from build123d import *

# Parameters (mm, degrees)
REDONDEO1_R = 1


with BuildPart() as part:
    # Croquis1 → Revolución1 (revolve)
    with BuildSketch(Plane.XY, mode=Mode.PRIVATE) as revoluci_n1_sk:
        Polygon((0, 2.465), (9.82, 2.465), (9.82, 6.5), (3, 6.5), (3, 8), (0, 8), align=None)
    revolve(revoluci_n1_sk.sketch.rotate(Axis((0, 0, 0), (1, 0, 0)), 90), axis=Axis((0, 0, 0), (1, 0, 0)))

    # Redondeo1
    redondeo1_edges = [part.edges().sort_by_distance(p)[0] for p in [
        (0, 0, -8),
        (9.82, 0, -6.5),
    ]]
    fillet(redondeo1_edges, radius=REDONDEO1_R)


solid = part.part
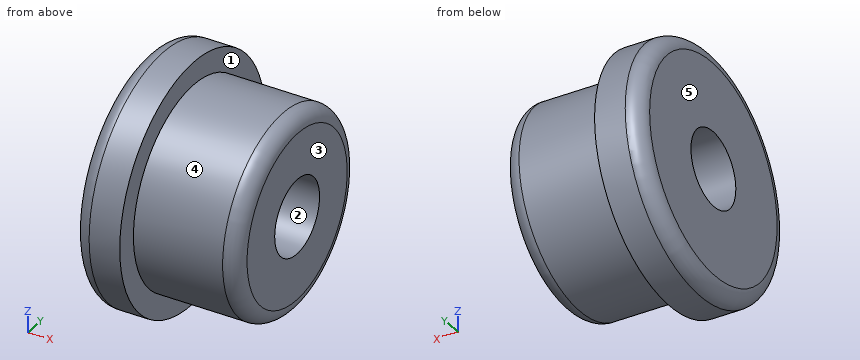
Geometry: final body of the model. Coordinates: model frame, mm. Face numbers are marked on the shaded views. A direction names the side the tool comes from. Coordinates: 2 decimals unless noted, no trailing zeros. Loops run counter-clockwise (first coordinate to the right, second up) from the corner with the lowest first, then second, coordinate; pieces in that order, holes last. Notation, with made-up numbers: M 61,-34 L 86,-34 A30 cw 86,-7 Z; hole C 21.25,80.25 d7. An arc over 180 degrees is marked long. One line per item, written item: value. Start each with the question number.
1) Cut plane A-A (z = 0). Return loops of the section in (x, y) (3 decimals).
2) Reachability of the marked faces 1 and 2 from +Z, -Z, +X, -X, +Y, -Y: full face, straight path, thin tool, end or side. Return the list, or none.
3) Pin query (flat end, axial travel): P1, Ø3, axis at y = 5, z = 1, coming from the -X side; P2, Ø4, axis at x = 6.5, z = -3, coming from the +Y side; P3, Ø1.5, axis at x = 8.5, y = -2.5, coming from the +Z side; P4, Ø4, axis at x = 3, y = -3.5, coming from the +Z side. Return the tip coordinate at first contact, or that it passes through.
4) Draft query along X for the marked faces 3, 4 and 5. Return one class per face: released by +X, released by -X, zero draft, split by the parting line, or undercut.
5) Cut plane C-C (x = 2.5). Return loops of the section in (y, z) (3 decimals), then the cut area to 3 significant figures.
6) Cut plane D-D (x = 0.5). Return loops of the section in (y, z) (3 decimals), then the cut area to 3 significant figures.
7) Material intervals for L1, parallel to Y at x = 7.25, z = 0 (3 decimals); L2, parallel to Y at x = 1.75, z = 0 (3 decimals); L3, parallel to X at y = 2.5, z = -5, sorted ascending. Write a range as from..to.
Evaluation:
1. outline: M 0,-7 A1 ccw 1,-8 L 3,-8 L 3,-6.5 L 8.82,-6.5 A1 ccw 9.82,-5.5 L 9.82,-2.465 L 0,-2.465 Z; M 0,2.465 L 9.82,2.465 L 9.82,5.5 A1 ccw 8.82,6.5 L 3,6.5 L 3,8 L 1,8 A1 ccw 0,7 Z
2. face 1: +X
2. face 2: +X, -X
3. P1: x = 0
3. P2: y = 6.42
3. P3: z = 6.26
3. P4: z = 7.86
4. face 3: released by +X
4. face 4: zero draft
4. face 5: released by -X
5. outline: C 0,0 d16; hole C 0,0 d4.93
5. area: 182 mm^2
6. outline: C 0,0 d15.732; hole C 0,0 d4.93
6. area: 175 mm^2
7. L1: -6.5..-2.465, 2.465..6.5
7. L2: -8..-2.465, 2.465..8
7. L3: 0..9.82
